from build123d import *

# Parameters (mm, degrees)
SKETCH1_W           = 90
SKETCH1_H           = 50
BOSS_EXTRUDE1_DEPTH = 90
SKETCH2_R           = 7.65
CUT_EXTRUDE1_DEPTH  = 104.682206767
SKETCH3_R           = 2.25
CUT_EXTRUDE2_DEPTH  = 10
SKETCH4_R           = 1.5
CUT_EXTRUDE3_DEPTH  = 10
SKETCH5_R           = 1.5
CUT_EXTRUDE4_DEPTH  = 104.682206767
CHAMFER1_SIZE       = 1
SKETCH6_W           = 23
SKETCH6_H           = 25
CUT_EXTRUDE5_DEPTH  = 104.682206767
CHAMFER2_SIZE       = 1


with BuildPart() as part:
    # Sketch1 → Boss-Extrude1 (new body)
    with BuildSketch(Plane.XY):
        Rectangle(SKETCH1_W, SKETCH1_H)
    extrude(amount=BOSS_EXTRUDE1_DEPTH)

    # Sketch2 → Cut-Extrude1 (cut, through all)
    with BuildSketch(Plane.XY.offset(90)):
        with Locations((-30, 0)):
            Circle(SKETCH2_R)
        with Locations((30, 0)):
            Circle(SKETCH2_R)
    extrude(amount=-CUT_EXTRUDE1_DEPTH, mode=Mode.SUBTRACT)

    # Sketch3 → Cut-Extrude2 (cut)
    with BuildSketch(Plane.ZY.offset(45)):
        with Locations(Location((20, 20, 0), (0, 0, 270))):
            Circle(SKETCH3_R)
        with Locations(Location((70, 20, 0), (0, 0, 90))):
            Circle(SKETCH3_R)
    extrude(amount=-CUT_EXTRUDE2_DEPTH, mode=Mode.SUBTRACT)

    # Sketch4 → Cut-Extrude3 (cut)
    with BuildSketch(Plane.XZ.offset(25)):
        with Locations(Location((-38, 70, 0), (0, 0, 270))):
            Circle(SKETCH4_R)
        with Locations(Location((-38, 20, 0), (0, 0, 270))):
            Circle(SKETCH4_R)
    extrude(amount=-CUT_EXTRUDE3_DEPTH, mode=Mode.SUBTRACT)

    # Sketch5 → Cut-Extrude4 (cut, through all)
    with BuildSketch(Plane.XY.offset(90)):
        with Locations((-38.485281374, 8.485281374)):
            Circle(SKETCH5_R)
        with Locations((-21.514718626, 8.485281374)):
            Circle(SKETCH5_R)
        with Locations((-21.514718626, -8.485281374)):
            Circle(SKETCH5_R)
        with Locations((-38.485281374, -8.485281374)):
            Circle(SKETCH5_R)
        with Locations((38.485281374, -8.485281374)):
            Circle(SKETCH5_R)
        with Locations((21.514718626, -8.485281374)):
            Circle(SKETCH5_R)
        with Locations((21.514718626, 8.485281374)):
            Circle(SKETCH5_R)
        with Locations((38.485281374, 8.485281374)):
            Circle(SKETCH5_R)
    extrude(amount=-CUT_EXTRUDE4_DEPTH, mode=Mode.SUBTRACT)

    # Chamfer1
    chamfer1_edges = [part.edges().sort_by_distance(p)[0] for p in [
        (-45, 0, 90),
        (0, -25, 90),
        (45, 0, 90),
        (0, -25, 0),
        (-45, 0, 0),
        (0, 25, 0),
        (45, 0, 0),
        (45, -25, 45),
        (-45, -25, 45),
        (-45, 25, 45),
        (45, 25, 45),
        (0, 25, 90),
    ]]
    chamfer(chamfer1_edges, length=CHAMFER1_SIZE)

    # Sketch6 → Cut-Extrude5 (cut, through all)
    with BuildSketch(Plane.XY.offset(90)):
        with Locations((3.5, 2)):
            Rectangle(SKETCH6_W, SKETCH6_H)
    extrude(amount=-CUT_EXTRUDE5_DEPTH, mode=Mode.SUBTRACT)

    # Chamfer2
    chamfer2_edges = [part.edges().sort_by_distance(p)[0] for p in [
        (15, 14.5, 45),
        (15, -10.5, 45),
        (-8, -10.5, 45),
        (-8, 14.5, 45),
    ]]
    chamfer(chamfer2_edges, length=CHAMFER2_SIZE)


solid = part.part
Verification items for the finished model (mm, model axes). A direction names the side the tool comes from. Coordinates: 2 decimals unless noted, no trailing zeros. Write each loop counter-clockwise with the first axis right and the second up, starting at its lowest first coordinate (ties: lowest second). Pieces come first, ordered by that corner, then holes. Notation, with made-up numbers: M -26.5,-5.5 L 28.5,-5.5 A6 cw 28.5,2.5 Z; hole C 65.5,42 d8. An arc over 180 degrees is marked long. Use a Markdown table: item, result.
Q1. Sectioned sample at A-A, the plane x = 30. Record the boundary of the cut face in (y, z), plus the area to 3 significant figures.
Reply:
| item | result |
|---|---|
| outline | M -25,1 L -24,0 L -7.65,0 L -7.65,90 L -24,90 L -25,89 Z; M 7.65,0 L 24,0 L 25,1 L 25,89 L 24,90 L 7.65,90 Z |
| area | 3,120 mm² |
Q2. Thickness scan on line 1 (X direction, y = 11, z = 22.5); line 2 (Y direction, x = -30.5, z = 6); line 3 (Y direction, x = -41.5, z = 70). Record the ranges inside material, lowest first.
Reply:
| item | result |
|---|---|
| line 1 | x = -45 to -8, 15 to 45 |
| line 2 | y = -25 to -7.63, 7.63 to 25 |
| line 3 | y = -25 to 17.75, 22.25 to 25 |
Q3. Sectioned sample at B-B, the plane y = 0. Record the boundary of the cut face in (x, z).
Reply:
| item | result |
|---|---|
| outline | M -45,1 L -44,0 L -37.65,0 L -37.65,90 L -44,90 L -45,89 Z; M -22.35,0 L -8,0 L -8,90 L -22.35,90 Z; M 15,0 L 22.35,0 L 22.35,90 L 15,90 Z; M 37.65,0 L 44,0 L 45,1 L 45,89 L 44,90 L 37.65,90 Z |
Q4. Sectioned sample at C-C, the plane z = 57. Count the separate pieces of the cut face and the enclosed holes in it, plus the area to 3 significant figures.
Reply:
| item | result |
|---|---|
| separate pieces | 1 |
| enclosed holes | 11 |
| area | 3,500 mm² |
Q5. Draft check along X on faces 1 (the face through (-40.07, 18.962, 18.004)), 2 (the face through (36.987, 8.551, 45.63)), 3 (the face through (-35, 20, 70)). Enter one of: +X half, -X half, draft (parallel to the pull), parting line (faces both ways), or undercut.
Reply:
| item | result |
|---|---|
| face 1 | draft |
| face 2 | undercut |
| face 3 | -X half |
Q6. Go/stop test with a flat-tipped pin: P1, Ø4, axis at x = -38.49, y = 8.49, coming from the +Z side. Record where the tip stops, or that it passes through.
Reply:
| item | result |
|---|---|
| P1 | stops at z = 90 |
Q7. Set-up check for faces 4 (the face through (-38.9, -20.1, 21.2)), 5 (the face through (3, 14.5, 46)), 6 (the face through (-35, 20, 20)), 7 (the face through (-45, 0, 44)): record each of +Z, -Z, +X, -X, +Y, -Y from which the full face is reachable in a straight line by a thin tool's end or side.
Reply:
| item | result |
|---|---|
| face 4 | -Y |
| face 5 | +Z, -Z |
| face 6 | -X |
| face 7 | +Z, -Z, -X, +Y, -Y |
